Check sheet for the modelled part. Datum: model origin and axes. Units: mm. Face numbers are marked on the shaded views. A direction names the side the tool comes from. Give positions to 0.01 mm unless a question says otherwise; leave off trailing zeros. Order: outer loops, then holes, each group sorted by start corner. A loop starts at its lowest first (then second) coordinate and runs counter-clockwise, first axis right, second up.
Item 1: Sectioned sample at C-C on y = 0. Record the boundary of the cut face in (x, z), and give its area (3 significant figures).
Item 2: Material ranges on line 1 along Y through (x, z) = (12.15, -16); line 2 along Y through (x, z) = (-9.75, 11); line 3 along X through (y, z) = (0.75, -8.5), recorded low to high.
Item 3: Access from +Z, -Z, +X, -X, +Y, -Y to the whole of each face (thin tool, end or side, straight path). Record for the marked faces 1, 2 and 3.
Item 4: Sectioned sample at B-B on z = 15. Record the boundary of the cut face in (x, y), and give its area (3 significant figures).
Item 5: Gauge pin test, flat end, axial feed: P1, Ø1, axis at x = -6.5, y = -8.5, coming from the +Z side. Record the tip position at first contact, or that the pin passes through.
Item 6: Sectioned sample at A-A on z = 23.5. Record the boundary of the cut face in (x, y).
Item 7: Sectioned sample at D-D on x = -8.5. Record the boundary of the cut face in (y, z).
Item 8: Release check for a two-part mould opening along X. For the marked faces 4, 5 and 6 record: released by +X, released by -X, zero draft, split by the parting line, or undercut.
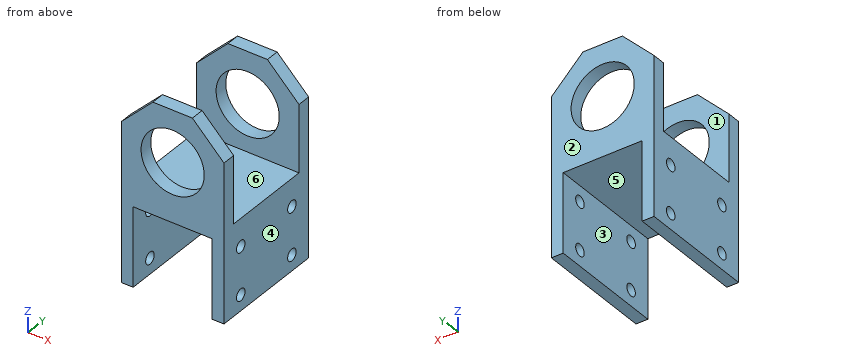
from build123d import *

# Parameters (mm, degrees)
SKETCH_1_W           = 26
SKETCH_1_H           = 20
EXTRUDE_1_DEPTH      = 3
EXTRUDE_2_DEPTH      = 16
SKETCH_5_W           = 3
SKETCH_5_H           = 20
EXTRUDE_3_DEPTH      = 20
SKETCH_8_W           = 23
SKETCH_8_H           = 8
CUT_EXTRUDE_5_DEPTH  = 40
CHAMFER_1_SIZE       = 8
SKETCH_16_W          = 23
SKETCH_16_H          = 4
CUT_EXTRUDE_8_DEPTH  = 26
SKETCH_17_W          = 16.892856711
SKETCH_17_H          = 8
CUT_EXTRUDE_9_DEPTH  = 10
EXTRUDE_4_DEPTH      = 14
CUT_EXTRUDE_10_DEPTH = 14
SKETCH_20_R          = 8
CUT_EXTRUDE_11_DEPTH = 39
SKETCH_21_R          = 9
CUT_EXTRUDE_12_DEPTH = 0.1
CUT_EXTRUDE_START    = -0.1
SKETCH_22_R          = 9
CUT_EXTRUDE_13_DEPTH = 0.1
SKETCH_23_R          = 1.5
CUT_EXTRUDE_14_DEPTH = 38.1
CUT_EXTRUDE_15_DEPTH = 0.5
CUT_EXTRUDE_16_DEPTH = 0.5
CUT_EXTRUDE_17_DEPTH = 0.1
CUT_EXTRUDE_18_DEPTH = 0.1


with BuildPart() as part:
    # 草图1 → 凸台-拉伸1 (new body)
    with BuildSketch(Plane.XY):
        Rectangle(SKETCH_1_W, SKETCH_1_H)
    extrude(amount=EXTRUDE_1_DEPTH)

    # 草图2 → 凸台-拉伸2 (add)
    with BuildSketch(Plane.XZ.offset(10)):
        Polygon((-13, 3), (-13, 15), (-13, 28), (13, 28), (13, 15), (13, 3), align=None)
    extrude(amount=-EXTRUDE_2_DEPTH)

    # 草图5 → 凸台-拉伸3 (add)
    with BuildSketch(Plane(origin=(0, 0, 0), x_dir=(-1, 0, 0), z_dir=(0, 0, -1))):
        with Locations((11.5, 0)):
            Rectangle(SKETCH_5_W, SKETCH_5_H)
        with Locations((-11.5, 0)):
            Rectangle(SKETCH_5_W, SKETCH_5_H)
    extrude(amount=EXTRUDE_3_DEPTH)

    # 草图8 → 切除-拉伸5 (cut)
    with BuildSketch(Plane(origin=(13, 0, 0), x_dir=(0, 0, -1), z_dir=(1, 0, 0))):
        with Locations((-14.5, -2)):
            Rectangle(SKETCH_8_W, SKETCH_8_H)
    extrude(amount=-CUT_EXTRUDE_5_DEPTH, mode=Mode.SUBTRACT)

    # 倒角1
    # the kernel refuses this chamfer: 8 mm, written as the material it takes off along each edge
    with BuildSketch(Plane(origin=(-13, -30.573463904, 28), x_dir=(-0.02749587661058627, 0, -0.9996219169112968), z_dir=(0, 1, 0)), Plane(origin=(13, -30.573463904, 28), x_dir=(-0.9996219169112968, 0, 0.027495876610586487), z_dir=(0, 1, 0))) as chamfer_1_piece_1:
        Polygon((CHAMFER_1_SIZE * 0.999621916911, -CHAMFER_1_SIZE * 0.0274958766106), (-CHAMFER_1_SIZE * 0.0274958766106, -CHAMFER_1_SIZE * 0.999621916911), (0, 0), align=None)
    extrude(amount=57.146927807, mode=Mode.SUBTRACT)

    # 草图16 → 切除-拉伸8 (cut)
    with BuildSketch(Plane(origin=(13, 0, 0), x_dir=(0, 0, -1), z_dir=(1, 0, 0))):
        with Locations((8.5, 8)):
            Rectangle(SKETCH_16_W, SKETCH_16_H)
    extrude(amount=-CUT_EXTRUDE_8_DEPTH, mode=Mode.SUBTRACT)

    # 草图17 → 切除-拉伸9 (cut)
    with BuildSketch(Plane.XY.offset(28)):
        with Locations((0.093159136, -2)):
            Rectangle(SKETCH_17_W, SKETCH_17_H)
    extrude(amount=-CUT_EXTRUDE_9_DEPTH, mode=Mode.SUBTRACT)

    # 草图18 → 凸台-拉伸4 (add)
    with BuildSketch(Plane.XZ.offset(10)):
        Polygon((5, 28), (-5, 28), (-13, 20), (-13, -20), (-10, -20), (-10, 0), (10, 0), (10, -20), (13, -20), (13, 20), align=None)
    extrude(amount=EXTRUDE_4_DEPTH)

    # 草图19 → 切除-拉伸10 (cut)
    with BuildSketch(Plane(origin=(0, -6, 0), x_dir=(1, 0, 0), z_dir=(0, 1, 0))):
        Polygon((5, -28), (13, -20), (13, -3), (-13, -3), (-13, -20), (-5, -28), align=None)
    extrude(amount=-CUT_EXTRUDE_10_DEPTH, mode=Mode.SUBTRACT)

    # 草图20 → 切除-拉伸11 (cut)
    with BuildSketch(Plane.XZ.offset(24)):
        with Locations(Location((0, 15, 0), (0, 0, 270))):
            Circle(SKETCH_20_R)
    extrude(amount=-CUT_EXTRUDE_11_DEPTH, mode=Mode.SUBTRACT)

    # 草图21 → 切除-拉伸12 (cut)
    with BuildSketch(Plane.XZ.offset(24)):
        with Locations(Location((0, 15, 0), (0, 0, 270))):
            Circle(SKETCH_21_R)
    extrude(amount=-CUT_EXTRUDE_12_DEPTH, mode=Mode.SUBTRACT)

    # 草图22 → 切除-拉伸13 (cut)
    with BuildSketch(Plane(origin=(0, 6, 0), x_dir=(1, 0, 0), z_dir=(0, 1, 0)).offset(CUT_EXTRUDE_START)):
        with Locations(Location((0, -15, 0), (0, 0, 90))):
            Circle(SKETCH_22_R)
    extrude(amount=CUT_EXTRUDE_13_DEPTH, mode=Mode.SUBTRACT)

    # 草图23 → 切除-拉伸14 (cut)
    with BuildSketch(Plane(origin=(13, 0, 0), x_dir=(0, 0, -1), z_dir=(1, 0, 0))):
        with Locations((4, 0)):
            Circle(SKETCH_23_R)
        with Locations((16, 0)):
            Circle(SKETCH_23_R)
        with Locations((4, -18)):
            Circle(SKETCH_23_R)
        with Locations((16, -18)):
            Circle(SKETCH_23_R)
    extrude(amount=-CUT_EXTRUDE_14_DEPTH, mode=Mode.SUBTRACT)

    # 草图24 → 切除-拉伸15 (cut)
    with BuildSketch(Plane.XZ.offset(-2)):
        Polygon((-5, 28), (-13, 20), (-13, 3), (13, 3), (13, 20), (5, 28), align=None)
    extrude(amount=-CUT_EXTRUDE_15_DEPTH, mode=Mode.SUBTRACT)

    # 草图25 → 切除-拉伸16 (cut)
    with BuildSketch(Plane(origin=(0, -20, 0), x_dir=(1, 0, 0), z_dir=(0, 1, 0))):
        Polygon((-5, -28), (5, -28), (13, -20), (13, -3), (-13, -3), (-13, -20), align=None)
    extrude(amount=-CUT_EXTRUDE_16_DEPTH, mode=Mode.SUBTRACT)

    # 草图26 → 切除-拉伸17 (cut)
    with BuildSketch(Plane.XZ.offset(24)):
        Polygon((13, 20), (5, 28), (-5, 28), (-13, 20), (-13, -20), (-10, -20), (-10, 0), (10, 0), (10, -20), (13, -20), align=None)
    extrude(amount=-CUT_EXTRUDE_17_DEPTH, mode=Mode.SUBTRACT)

    # 草图27 → 切除-拉伸18 (cut)
    with BuildSketch(Plane(origin=(0, 6, 0), x_dir=(1, 0, 0), z_dir=(0, 1, 0))):
        Polygon((-13, 20), (-13, -20), (-5, -28), (5, -28), (13, -20), (13, 20), (10, 20), (10, 0), (-10, 0), (-10, 20), align=None)
    extrude(amount=-CUT_EXTRUDE_18_DEPTH, mode=Mode.SUBTRACT)


solid = part.part
Report:
1. outline: (-13, -20) - (-10, -20) - (-10, -17.5) - (-13, -17.5) - close; (-13, -14.5) - (-10, -14.5) - (-10, -5.5) - (-13, -5.5) - close; (-13, -2.5) - (-10, -2.5) - (-10, 0) - (10, 0) - (10, -2.5) - (13, -2.5) - (13, 3) - (-13, 3) - close; (10, -20) - (13, -20) - (13, -17.5) - (10, -17.5) - close; (10, -14.5) - (13, -14.5) - (13, -5.5) - (10, -5.5) - close
1. area: 162 mm2
2. line 1: y = -23.9 to -19.5, -16.5 to -1.5, 1.5 to 5.9
2. line 2: y = -23.9 to -20.5, 2.5 to 5.9
2. line 3: x = -13 to -10, 10 to 13
3. face 1: +Z, +X, -X
3. face 2: +Z, -Z, +X, -X, +Y
3. face 3: -Z, +Y, -Y
4. outline: (-13, -23.9) - (-8, -23.9) - (-8, -20.5) - (-13, -20.5) - close; (-13, 2.5) - (-8, 2.5) - (-8, 5.9) - (-13, 5.9) - close; (8, -23.9) - (13, -23.9) - (13, -20.5) - (8, -20.5) - close; (8, 2.5) - (13, 2.5) - (13, 5.9) - (8, 5.9) - close
4. area: 68.0 mm2
5. P1: stops at z = 3
6. outline: (-9.5, -23.9) - (9.5, -23.9) - (9.5, -20.5) - (-9.5, -20.5) - close; (-9.5, 2.5) - (9.5, 2.5) - (9.5, 5.9) - (-9.5, 5.9) - close
7. outline: (-23.9, 0) - (5.9, 0) - (5.9, 24.5) - (2.5, 24.5) - (2.5, 3) - (-20.5, 3) - (-20.5, 24.5) - (-23.9, 24.5) - close
8. face 4: released by +X
8. face 5: undercut
8. face 6: zero draft
